Here's how the part is built. I have some questions about the finished solid (model axes, mm). A direction names the side the tool comes from. Round coordinates to 2 decimals unless told otherwise and drop trailing zeros. Loops run counter-clockwise (first coordinate to the right, second up) from the corner with the lowest first, then second, coordinate; pieces in that order, holes last. Notation, with made-up numbers: M 49,-19.75 L 69,-19.75 A28 cw 69,19.25 Z; hole C -0.75,63.25 d1. An arc over 180 degrees is marked long. Answer as a JSON object with one key per item and string values.
from build123d import *

# Parameters (mm, degrees)
SKETCH2_R           = 11.95
BOSS_EXTRUDE1_DEPTH = 30.4
SKETCH4_R           = 1.5
CUT_EXTRUDE2_DEPTH  = 3
SKETCH5_R           = 0.99
BOSS_EXTRUDE2_DEPTH = 6.9


with BuildPart() as part:
    # Sketch2 → Boss-Extrude1 (new body)
    with BuildSketch(Plane.XY):
        Circle(SKETCH2_R)
    extrude(amount=BOSS_EXTRUDE1_DEPTH)

    # Sketch4 → Cut-Extrude2 (cut)
    with BuildSketch(Plane(origin=(0, 0, 0), x_dir=(-1, 0, 0), z_dir=(0, 0, -1))):
        with Locations((0, 8.95)):
            Circle(SKETCH4_R)
        with Locations((0, -8.95)):
            Circle(SKETCH4_R)
    extrude(amount=-CUT_EXTRUDE2_DEPTH, mode=Mode.SUBTRACT)

    # Sketch5 → Boss-Extrude2 (add)
    with BuildSketch(Plane(origin=(0, 0, 0), x_dir=(-1, 0, 0), z_dir=(0, 0, -1))):
        Circle(SKETCH5_R)
    extrude(amount=BOSS_EXTRUDE2_DEPTH)


solid = part.part
Item 1: I want a section at D-D, the plane y = -8.95. Please give me the cut outline in (x, z), then the cut area to 3 significant figures.
Resolved:
{"outline": "M -7.92,0 L -1.5,0 L -1.5,3 L 1.5,3 L 1.5,0 L 7.92,0 L 7.92,30.4 L -7.92,30.4 Z", "area": "472 mm²"}
Item 2: I want a section at C-C, the plane z = 15. Please give me the cut outline in (x, y), then the cut area to 3 significant figures.
Resolved:
{"outline": "C 0,0 d23.9", "area": "449 mm²"}
Item 3: I want a section at A-A, the plane x = 0. Please give me the cut outline in (y, z), then the cut area to 3 significant figures.
Resolved:
{"outline": "M -11.95,0 L -10.45,0 L -10.45,3 L -7.45,3 L -7.45,0 L -0.99,0 L -0.99,-6.9 L 0.99,-6.9 L 0.99,0 L 7.45,0 L 7.45,3 L 10.45,3 L 10.45,0 L 11.95,0 L 11.95,30.4 L -11.95,30.4 Z", "area": "722 mm²"}
Item 4: If we mould it in two halves opening along Y, with no side actions, what happens to faces 1 (the face through (0, 0, -6.9)), 2 (the face through (0.215, -0.966, -3.402)), 3 (the face through (0.325, -10.414, 1.479))? For each: pulls with the +Y half, pulls with the -Y half, needs draft (parallel to the pull), parting line crosses it, or undercut.
Resolved:
{"face 1": "needs draft", "face 2": "parting line crosses it", "face 3": "undercut"}
Item 5: On a 3-axis mill with a long thin cutter (end or side, diameter ignored), from which of +Z, -Z, +X, -X, +Y, -Y can I reach the whole of each face in a straight line? I mean faces 4 (the face through (0, 9, 3)), 5 (the face through (6.42, 10.08, 14.99)). Say none if no direction works.
Resolved:
{"face 4": "-Z", "face 5": "+Z, -Z"}
Item 6: I want a section at B-B, the plane y = 0. Please give me the cut outline in (x, z).
Resolved:
{"outline": "M -11.95,0 L -0.99,0 L -0.99,-6.9 L 0.99,-6.9 L 0.99,0 L 11.95,0 L 11.95,30.4 L -11.95,30.4 Z"}
Item 7: Please list where these lines run through material, in increasing order: probe 1 along Y at (x, z) = (0, 0.8); probe 2 along Z at (x, y) = (3.25, -7); probe 3 along Y at (x, z) = (1.25, 10). Write a range as from..to.
Resolved:
{"probe 1": "-11.95..-10.45, -7.45..7.45, 10.45..11.95", "probe 2": "0..30.4", "probe 3": "-11.88..11.88"}
Item 8: I'm going to push flat-ended pins straight in: pin 1 Ø3.5 at (x, y) = (0, -8.5) entering from -Z; pin 2 Ø1.5 at (x, z) = (-1.5, 7) entering from -Y; pin 3 Ø5 at (y, z) = (9.5, 16) entering from +X; pin 4 Ø10 at (x, z) = (-3.5, 25) entering from +Y. Where does each tip first touch, or does it pass through?
Resolved:
{"pin 1": "z = 0", "pin 2": "y = -11.93", "pin 3": "x = 9.69", "pin 4": "y = 11.95"}
